```python
from build123d import *

# Parameters (mm, degrees)
SKETCH1_W           = 162.56
SKETCH1_H           = 12.7
BOSS_EXTRUDE1_DEPTH = 15.24
SKETCH2_R           = 1.8034
CUT_EXTRUDE1_DEPTH  = 15.24
SKETCH3_R           = 5.1181
CUT_EXTRUDE2_DEPTH  = 15.24
SKETCH4_W           = 8.89
SKETCH4_H           = 15.24
BOSS_EXTRUDE2_DEPTH = 57.15
FILLET1_R           = 5.08
SKETCH5_R           = 1.6256
SKETCH5_R_2         = 1.8034
CUT_EXTRUDE3_DEPTH  = 152.4
SKETCH6_R           = 4.3815
CUT_EXTRUDE4_DEPTH  = 1.27
SKETCH7_R           = 3.2639
CUT_EXTRUDE5_DEPTH  = 2.54
SKETCH8_W           = 39.37
SKETCH8_H           = 7.62
CUT_EXTRUDE6_DEPTH  = 25.4
FILLET2_R           = 1.27
FILLET3_R           = 1.27


with BuildPart() as part:
    # Sketch1 → Boss-Extrude1 (new body)
    with BuildSketch(Plane.XY):
        Rectangle(SKETCH1_W, SKETCH1_H)
    extrude(amount=BOSS_EXTRUDE1_DEPTH)

    # Sketch2 → Cut-Extrude1 (cut)
    with BuildSketch(Plane(origin=(0, 0, 0), x_dir=(-1, 0, 0), z_dir=(0, 0, -1))):
        with Locations((-76.2, 0)):
            Circle(SKETCH2_R)
        with Locations((-57.15, 0)):
            Circle(SKETCH2_R)
        with Locations((57.15, 0)):
            Circle(SKETCH2_R)
        with Locations((76.2, 0)):
            Circle(SKETCH2_R)
    extrude(amount=-CUT_EXTRUDE1_DEPTH, mode=Mode.SUBTRACT)

    # Sketch3 → Cut-Extrude2 (cut)
    with BuildSketch(Plane(origin=(0, 0, 0), x_dir=(-1, 0, 0), z_dir=(0, 0, -1))):
        Circle(SKETCH3_R)
    extrude(amount=-CUT_EXTRUDE2_DEPTH, mode=Mode.SUBTRACT)

    # Sketch4 → Boss-Extrude2 (add)
    with BuildSketch(Plane(origin=(0, 6.35, 0), x_dir=(1, 0, 0), z_dir=(0, 1, 0))):
        with Locations((67.78498, -7.62)):
            Rectangle(SKETCH4_W, SKETCH4_H)
        with Locations((-67.78752, -7.62)):
            Rectangle(SKETCH4_W, SKETCH4_H)
    extrude(amount=BOSS_EXTRUDE2_DEPTH)

    # Fillet1
    fillet1_edges = [part.edges().sort_by_distance(p)[0] for p in [
        (72.22998, 6.35, 7.62),
        (63.33998, 6.35, 7.62),
        (-63.34252, 6.35, 7.62),
        (-72.23252, 6.35, 7.62),
    ]]
    fillet(fillet1_edges, radius=FILLET1_R)

    # Sketch5 → Cut-Extrude3 (cut)
    with BuildSketch(Plane(origin=(72.22998, 0, 0), x_dir=(0, 0, -1), z_dir=(1, 0, 0))):
        with Locations((-7.62, 60.325)):
            Circle(SKETCH5_R)
        with Locations((-7.62, 34.925)):
            Circle(SKETCH5_R)
        with Locations((-7.62, 47.625)):
            Circle(SKETCH5_R_2)
    extrude(amount=-CUT_EXTRUDE3_DEPTH, mode=Mode.SUBTRACT)

    # Sketch6 → Cut-Extrude4 (cut)
    with BuildSketch(Plane(origin=(72.22998, 0, 0), x_dir=(0, 0, -1), z_dir=(1, 0, 0))):
        with Locations((-7.62, 47.625)):
            Circle(SKETCH6_R)
    extrude(amount=-CUT_EXTRUDE4_DEPTH, mode=Mode.SUBTRACT)

    # Sketch7 → Cut-Extrude5 (cut)
    with BuildSketch(Plane.ZY.offset(72.23252)):
        with Locations((7.62, 47.625)):
            Circle(SKETCH7_R)
    extrude(amount=-CUT_EXTRUDE5_DEPTH, mode=Mode.SUBTRACT)

    # Sketch8 → Cut-Extrude6 (cut)
    with BuildSketch(Plane(origin=(0, 6.35, 0), x_dir=(1, 0, 0), z_dir=(0, 1, 0))):
        with Locations((30.95498, -7.62)):
            Rectangle(SKETCH8_W, SKETCH8_H)
        with Locations((-30.95752, -7.62)):
            Rectangle(SKETCH8_W, SKETCH8_H)
    extrude(amount=-CUT_EXTRUDE6_DEPTH, mode=Mode.SUBTRACT)

    # Fillet2
    fillet2_edges = [part.edges().sort_by_distance(p)[0] for p in [
        (11.26998, 0, 11.43),
        (11.26998, 0, 3.81),
        (50.63998, 0, 3.81),
        (50.63998, 0, 11.43),
    ]]
    fillet(fillet2_edges, radius=FILLET2_R)

    # Fillet3
    fillet3_edges = [part.edges().sort_by_distance(p)[0] for p in [
        (-50.64252, 0, 11.43),
        (-50.64252, 0, 3.81),
        (-11.27252, 0, 3.81),
        (-11.27252, 0, 11.43),
    ]]
    fillet(fillet3_edges, radius=FILLET3_R)


solid = part.part
```
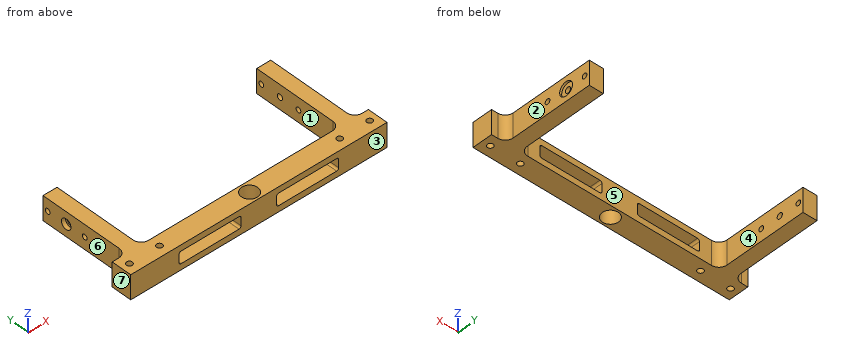
Input: part model. Units: mm. Frame: model coordinates. Face numbers are marked on the shaded views. A direction names the side the tool comes from. Give positions to 0.01 mm unless a question says otherwise; leave off trailing zeros. Loops run counter-clockwise (first coordinate to the right, second up) from the corner with the lowest first, then second, coordinate; pieces in that order, holes last. Notation, with made-up numbers: (22.25, 0) -> (75.25, 0) arc R20 cw to (75.25, 20) -> close; hole circle Ø3 at (67.25, 52). An arc over 180 degrees is marked (long way). Use a Markdown table: item, result.
Q1. Access query for the marked faces 5, 6 and 7. Directions: +Z, -Z, +X, -X, +Y, -Y. A direction counts if a zero-diameter tool reaches every point of the face in a straight line with its end or side. Return the directions, or none.
Entries:
| item | result |
|---|---|
| face 5 | +Z, -Z, +Y |
| face 6 | +Z, -Z, -X, +Y |
| face 7 | +Z, -Z, -X, +Y, -Y |
Q2. Pull-direction query (X, two-part tool) for the marked faces 1, 2, 3 and 4; classes: pulls with the +X half, pulls with the -X half, needs draft (parallel to the pull), parting line crosses it, or undercut.
Entries:
| item | result |
|---|---|
| face 1 | undercut |
| face 2 | pulls with the +X half |
| face 3 | needs draft |
| face 4 | undercut |
Q3. Section query B-B, the plane z = 13.5. Return the cut outline in (x, y), plus the area to 3 significant figures.
Entries:
| item | result |
|---|---|
| outline | (-81.28, -6.35) -> (81.28, -6.35) -> (81.28, 6.35) -> (77.31, 6.35) arc R5.08 cw to (72.23, 11.43) -> (72.23, 63.5) -> (63.34, 63.5) -> (63.34, 11.43) arc R5.08 cw to (58.26, 6.35) -> (-58.26, 6.35) arc R5.08 cw to (-63.34, 11.43) -> (-63.34, 63.5) -> (-72.23, 63.5) -> (-72.23, 11.43) arc R5.08 cw to (-77.31, 6.35) -> (-81.28, 6.35) -> close; hole circle Ø3.61 at (-76.2, 0); hole circle Ø3.61 at (-57.15, 0); hole circle Ø10.24 at (0, 0); hole circle Ø3.61 at (57.15, 0); hole circle Ø3.61 at (76.2, 0) |
| area | 2,980 mm² |
Q4. Section query D-D, the plane x = -61.5. Return the cut outline in (y, z).
Entries:
| item | result |
|---|---|
| outline | (-6.35, 0) -> (7.52, 0) -> (7.52, 15.24) -> (-6.35, 15.24) -> close |
Q5. First-contact query: P1, Ø4, axis at y = 47.625, z = 7.62, coming from the +X side; P2, Ø4, axis at y = 47.625, z = 7.62, coming from the -X side; P3, Ø3, axis at x = -76.2, y = 0, coming from the -Z side; P4, Ø4, axis at x = -0.5, z = 6.5, coming from the +Y side. Flat tips, straight axial feed; report the tip coordinate or a pass-through.
Entries:
| item | result |
|---|---|
| P1 | stops at x = 70.96 |
| P2 | stops at x = -69.69 |
| P3 | passes through |
| P4 | stops at y = 6.35 |
Q6. Section query A-A, the plane x = 0. Return the cut outline in (y, z).
Entries:
| item | result |
|---|---|
| outline | (-6.35, 0) -> (-5.12, 0) -> (-5.12, 15.24) -> (-6.35, 15.24) -> close; (5.12, 0) -> (6.35, 0) -> (6.35, 15.24) -> (5.12, 15.24) -> close |
Q7. Section query C-C, the plane x = -40.5. Return the cut outline in (y, z), plus the area to 3 significant figures.
Entries:
| item | result |
|---|---|
| outline | (-6.35, 0) -> (6.35, 0) -> (6.35, 3.81) -> (-6.35, 3.81) -> close; (-6.35, 11.43) -> (6.35, 11.43) -> (6.35, 15.24) -> (-6.35, 15.24) -> close |
| area | 96.8 mm² |
Q8. Ray query, probe 1 along Y at (x, z) = (70.25, 7.62); probe 2 along Z at (x, y) = (-19, 4); probe 3 along X at (y, z) = (19, 10.5). Return the intervals inside material, ascending. Write a range as from..to.
Entries:
| item | result |
|---|---|
| probe 1 | y = -6.35..33.3, 36.55..45.82, 49.43..58.7, 61.95..63.5 |
| probe 2 | z = 0..3.81, 11.43..15.24 |
| probe 3 | x = -72.23..-63.34, 63.34..72.23 |
